Part model, mm, in its own coordinate system. Face numbers are marked on the shaded views. A direction names the side the tool comes from. Round coordinates to 2 decimals unless told otherwise and drop trailing zeros. Loops run counter-clockwise (first coordinate to the right, second up) from the corner with the lowest first, then second, coordinate; pieces in that order, holes last. Notation, with made-up numbers: M 44,39 L 65,39 A19 cw 65,56 Z; hole C 16,-3 d8. An arc over 180 degrees is marked long. Put each result on its own line as item: value. Start each with the question number.
1) Drop flat-ended pins along their axis: pin 1 Ø1.8 at (y, z) = (5, 2) entering from -X; pin 2 Ø1.5 at (x, z) = (4, 5) entering from +Y; pin 3 Ø2 at (x, z) = (1, 2) entering from +Y; pin 4 Ø10 at (x, y) = (-7.5, -4) entering from -Z. Give the stop position or say it passes through.
2) Slice it at C-C on z = 5.75. Give the cut face in (x, y), then the cut area to 3 significant figures.
3) Probe line 1 along Z through (x, y) = (0, 8.3); line 2 along X through (y, z) = (7.7, 2.5); line 3 along Z through (x, y) = (-8.25, -6). List the from-to ranges inside material, lowest first.
4) Pull direction X, two halves, no side cores. Call the marked faces 1, 2, 3 and 4: +X half, -X half, draft (parallel to the pull), parting line (faces both ways), or undercut.
5) Which spindle directions (+Z, -Z, +X, -X, +Y, -Y) get a long thin tool onto all of the face, cutting with end or side? Do the marked faces 5 and 6. Say none if no direction does.
6) Slice it at B-B on x = -8. Give the cut face in (y, z).
7) Slice it at A-A on y = 0. Give the cut face in (x, z), then the cut area to 3 significant figures.
Autodesk Inventor part; units mm, degrees
ref_plane "YZ Plane" through (0, 0, 0) normal (1, 0, 0) x (0, 1, 0)
ref_plane "XY Plane" through (0, 0, 0) normal (0, 0, 1) x (1, 0, 0)
sketch "Sketch1" plane through (0, 0, 0) normal (0, 0, 1) x (1, 0, 0)
  circle A0 centre (0, 0) radius 9
  dimension "d0" = 18
extrude "Extrusion1" add sketch "Sketch1" along normal blind 5
sketch "Sketch2" plane through (0, 0, 5) normal (0, 0, 1) x (1, 0, 0)
  circle A0 centre (0, 0) radius 11
  circle A1 centre (0, 0) radius 9
  dimension "d3" = 2
extrude "Extrusion2" add sketch "Sketch2" along normal blind 1.6 contours A0 | A1
ref_plane "Work Plane1" through (0, 0, 2.5) normal (0, 0, 1) x (1, 0, 0)
sketch "Sketch3" plane through (0, 0, 2.5) normal (0, 0, 1) x (1, 0, 0)
  circle A0 centre (0, 0) radius 9
  point P0 (0, 9)
ref_plane "Work Plane2" through (0, 9, 2.5) normal (0, 1, 0) x (-1, 0, 0)
sketch "Sketch4" plane through (0, 9, 2.5) normal (0, 1, 0) x (-1, 0, 0)
  point P0 (0, -2.5)
  point P1 (0, 0)
hole "Hole1" at (0, 9, 2.5) direction (0, -1, 0) diameter 2.1 depth 6 tip angle 118
ref_plane "Work Plane3" through (0, 6, 2.5) normal (0, 1, 0) x (-1, 0, 0)
sketch "Sketch5" plane through (0, 6, 2.5) normal (0, 1, 0) x (-1, 0, 0)
  circle A0 centre (0, 0) radius 1.05
  line L0 (2.05, 1.1836) -> (2.05, -1.1836)
  line L1 (2.05, -1.1836) -> (0, -2.3671) construction
  line L2 (0, -2.3671) -> (-2.05, -1.1836) construction
  line L3 (-2.05, -1.1836) -> (-2.05, 1.1836)
  line L4 (-2.05, 1.1836) -> (0, 2.3671)
  line L5 (0, 2.3671) -> (2.05, 1.1836)
  line L6 (2.05, -1.1836) -> (2.05, -2.5)
  line L7 (9, -2.5) -> (-9, -2.5)
  line L8 (-2.05, -1.1836) -> (-2.05, -2.5)
  point P0 (0, -2.5)
  dimension "d14" = 4.1
extrude "Extrusion3" cut sketch "Sketch5" against normal blind 1.65
sketch "Sketch6" plane through (0, 0, 6.6) normal (0, 0, 1) x (1, 0, 0)
  circle A0 centre (0, 0) radius 3.0931 construction
hole "Hole3" at (0, 0, 6.6) direction (0, 0, -1) diameter 2.6 end through all
properties part number "Encoder_Mount3_Wheel"
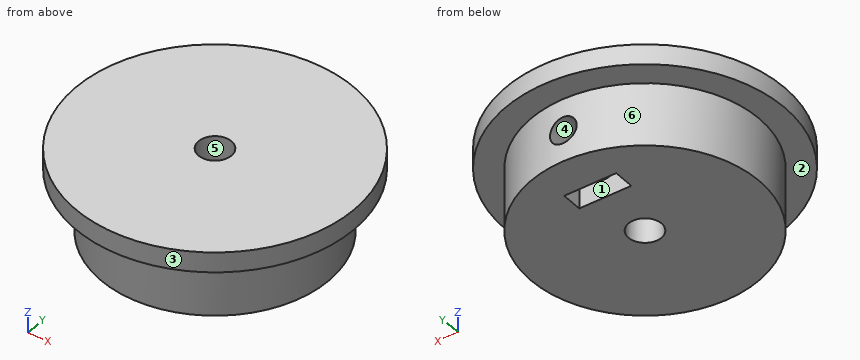
Recorded:
1. pin 1: stops at x = -8.01
1. pin 2: stops at y = 10.51
1. pin 3: stops at y = 9
1. pin 4: stops at z = 0
2. outline: C 0,0 d22; hole C 0,0 d2.6
2. area: 375 mm2
3. line 1: z = 0 to 1.45, 3.55 to 6.6
3. line 2: x = -4.66 to -1.05, 1.05 to 4.66
3. line 3: z = 5 to 6.6
4. face 1: undercut
4. face 2: draft
4. face 3: parting line
4. face 4: undercut
5. face 5: +Z, -Z
5. face 6: -Z
6. outline: M -7.55,5 L -4.12,5 L -4.12,0 L 4.12,0 L 4.12,5 L 7.55,5 L 7.55,6.6 L -7.55,6.6 Z
7. outline: M -11,5 L -9,5 L -9,0 L -1.3,0 L -1.3,6.6 L -11,6.6 Z; M 1.3,0 L 9,0 L 9,5 L 11,5 L 11,6.6 L 1.3,6.6 Z
7. area: 108 mm2
